```python
from build123d import *

# Parameters (mm, degrees)
PAD_DEPTH        = 44
SKETCH001_W      = 79.5
SKETCH001_H      = 39.5
POCKET_DEPTH     = 42
SKETCH003_W      = 79.5
SKETCH003_H      = 39.5
PAD001_DEPTH     = 11
SKETCH004_W      = 75.5
SKETCH004_H      = 35.5
POCKET001_DEPTH  = 11
HOLE_D           = 5.3
HOLE_DEPTH       = 25
HOLE_CSINK_D     = 6.1
HOLE_CSINK_ANGLE = 90
HOLE_TIPS_R      = 2.65
SKETCH056_W      = 7
SKETCH056_H      = 30
POCKET017_DEPTH  = 61.3
SKETCH054_W      = 7
SKETCH054_H      = 30
POCKET019_DEPTH  = 61.3
SKETCH057_W      = 12
SKETCH057_H      = 40
POCKET018_DEPTH  = 31
SKETCH055_W      = 12
SKETCH055_H      = 40
POCKET020_DEPTH  = 31
SKETCH005_W      = 15
SKETCH005_H      = 10
POCKET002_DEPTH  = 5
SKETCH058_W      = 81.5
SKETCH058_H      = 41.5
POCKET021_DEPTH  = 2
CHAMFER_SIZE     = 0.5
CHAMFER030_SIZE  = 0.3
CHAMFER031_SIZE  = 0.3


with BuildPart() as part:
    # Sketch → Pad (new body)
    with BuildSketch(Plane.XZ):
        with BuildLine():
            Line((99, 14), (99, -6))
            ThreePointArc((99, -6), (70.300448, -3.42122), (41.5, -2.5))
            Line((41.5, -21.5), (41.5, -2.5))
            ThreePointArc((-41.5, -21.5), (0, -23.225226), (41.5, -21.5))
            Line((-41.5, -2.5), (-41.5, -21.5))
            ThreePointArc((-41.5, -2.5), (-70.300448, -3.42122), (-99, -6))
            Line((-99, 14), (-99, -6))
            ThreePointArc((99, 14), (0, 23.89899), (-99, 14))
        make_face()
    extrude(amount=PAD_DEPTH)

    # Sketch001 (on DatumPlane) → Pocket (cut)
    with BuildSketch(Plane(origin=(0, 0, 0), x_dir=(1, 0, 0), z_dir=(0, 1, 0))):
        Rectangle(SKETCH001_W, SKETCH001_H)
    extrude(amount=-POCKET_DEPTH, mode=Mode.SUBTRACT)

    # Sketch003 → Pad001 (join)
    with BuildSketch(Plane(origin=(0, -42, 0), x_dir=(1, 0, 0), z_dir=(0, 1, 0))):
        Rectangle(SKETCH003_W, SKETCH003_H)
    extrude(amount=PAD001_DEPTH)

    # Sketch004 (on Face15 of Pad001) → Pocket001 (cut)
    with BuildSketch(Plane(origin=(0, -31, 0), x_dir=(1, 0, 0), z_dir=(0, 1, 0))):
        Rectangle(SKETCH004_W, SKETCH004_H)
    extrude(amount=-POCKET001_DEPTH, mode=Mode.SUBTRACT)

    # Hole
    with Locations(Plane.XZ.offset(44)):
        with Locations((-15.24, 11.43), (-7.62, 11.43), (0, 11.43), (7.62, 11.43), (15.24, 11.43), (-15.24, 3.81), (-7.62, 3.81), (0, 3.81), (7.62, 3.81), (15.24, 3.81), (-15.24, -3.81), (-7.62, -3.81), (0, -3.81), (7.62, -3.81), (15.24, -3.81), (-15.24, -11.43), (-7.62, -11.43), (0, -11.43), (7.62, -11.43), (15.24, -11.43)):
            CounterSinkHole(HOLE_D / 2, HOLE_CSINK_D / 2, depth=HOLE_DEPTH, counter_sink_angle=HOLE_CSINK_ANGLE)

    # Hole tips → Hole tip 1 section 0
    with BuildSketch(Plane.XZ.offset(19), mode=Mode.PRIVATE) as hole_tip_1_s0:
        with Locations((-15.24, 11.43)):
            Circle(HOLE_TIPS_R)
    loft([hole_tip_1_s0.sketch, Vertex(-15.24, -17.407719, 11.43)], mode=Mode.SUBTRACT)

    # Hole tips → Hole tip 2 section 0
    with BuildSketch(Plane.XZ.offset(19), mode=Mode.PRIVATE) as hole_tip_2_s0:
        with Locations((-7.62, 11.43)):
            Circle(HOLE_TIPS_R)
    loft([hole_tip_2_s0.sketch, Vertex(-7.62, -17.407719, 11.43)], mode=Mode.SUBTRACT)

    # Hole tips → Hole tip 3 section 0
    with BuildSketch(Plane.XZ.offset(19), mode=Mode.PRIVATE) as hole_tip_3_s0:
        with Locations((0, 11.43)):
            Circle(HOLE_TIPS_R)
    loft([hole_tip_3_s0.sketch, Vertex(0, -17.407719, 11.43)], mode=Mode.SUBTRACT)

    # Hole tips → Hole tip 4 section 0
    with BuildSketch(Plane.XZ.offset(19), mode=Mode.PRIVATE) as hole_tip_4_s0:
        with Locations((7.62, 11.43)):
            Circle(HOLE_TIPS_R)
    loft([hole_tip_4_s0.sketch, Vertex(7.62, -17.407719, 11.43)], mode=Mode.SUBTRACT)

    # Hole tips → Hole tip 5 section 0
    with BuildSketch(Plane.XZ.offset(19), mode=Mode.PRIVATE) as hole_tip_5_s0:
        with Locations((15.24, 11.43)):
            Circle(HOLE_TIPS_R)
    loft([hole_tip_5_s0.sketch, Vertex(15.24, -17.407719, 11.43)], mode=Mode.SUBTRACT)

    # Hole tips → Hole tip 6 section 0
    with BuildSketch(Plane.XZ.offset(19), mode=Mode.PRIVATE) as hole_tip_6_s0:
        with Locations((-15.24, 3.81)):
            Circle(HOLE_TIPS_R)
    loft([hole_tip_6_s0.sketch, Vertex(-15.24, -17.407719, 3.81)], mode=Mode.SUBTRACT)

    # Hole tips → Hole tip 7 section 0
    with BuildSketch(Plane.XZ.offset(19), mode=Mode.PRIVATE) as hole_tip_7_s0:
        with Locations((-7.62, 3.81)):
            Circle(HOLE_TIPS_R)
    loft([hole_tip_7_s0.sketch, Vertex(-7.62, -17.407719, 3.81)], mode=Mode.SUBTRACT)

    # Hole tips → Hole tip 8 section 0
    with BuildSketch(Plane.XZ.offset(19), mode=Mode.PRIVATE) as hole_tip_8_s0:
        with Locations((0, 3.81)):
            Circle(HOLE_TIPS_R)
    loft([hole_tip_8_s0.sketch, Vertex(0, -17.407719, 3.81)], mode=Mode.SUBTRACT)

    # Hole tips → Hole tip 9 section 0
    with BuildSketch(Plane.XZ.offset(19), mode=Mode.PRIVATE) as hole_tip_9_s0:
        with Locations((7.62, 3.81)):
            Circle(HOLE_TIPS_R)
    loft([hole_tip_9_s0.sketch, Vertex(7.62, -17.407719, 3.81)], mode=Mode.SUBTRACT)

    # Hole tips → Hole tip 10 section 0
    with BuildSketch(Plane.XZ.offset(19), mode=Mode.PRIVATE) as hole_tip_10_s0:
        with Locations((15.24, 3.81)):
            Circle(HOLE_TIPS_R)
    loft([hole_tip_10_s0.sketch, Vertex(15.24, -17.407719, 3.81)], mode=Mode.SUBTRACT)

    # Hole tips → Hole tip 11 section 0
    with BuildSketch(Plane.XZ.offset(19), mode=Mode.PRIVATE) as hole_tip_11_s0:
        with Locations((-15.24, -3.81)):
            Circle(HOLE_TIPS_R)
    loft([hole_tip_11_s0.sketch, Vertex(-15.24, -17.407719, -3.81)], mode=Mode.SUBTRACT)

    # Hole tips → Hole tip 12 section 0
    with BuildSketch(Plane.XZ.offset(19), mode=Mode.PRIVATE) as hole_tip_12_s0:
        with Locations((-7.62, -3.81)):
            Circle(HOLE_TIPS_R)
    loft([hole_tip_12_s0.sketch, Vertex(-7.62, -17.407719, -3.81)], mode=Mode.SUBTRACT)

    # Hole tips → Hole tip 13 section 0
    with BuildSketch(Plane.XZ.offset(19), mode=Mode.PRIVATE) as hole_tip_13_s0:
        with Locations((0, -3.81)):
            Circle(HOLE_TIPS_R)
    loft([hole_tip_13_s0.sketch, Vertex(0, -17.407719, -3.81)], mode=Mode.SUBTRACT)

    # Hole tips → Hole tip 14 section 0
    with BuildSketch(Plane.XZ.offset(19), mode=Mode.PRIVATE) as hole_tip_14_s0:
        with Locations((7.62, -3.81)):
            Circle(HOLE_TIPS_R)
    loft([hole_tip_14_s0.sketch, Vertex(7.62, -17.407719, -3.81)], mode=Mode.SUBTRACT)

    # Hole tips → Hole tip 15 section 0
    with BuildSketch(Plane.XZ.offset(19), mode=Mode.PRIVATE) as hole_tip_15_s0:
        with Locations((15.24, -3.81)):
            Circle(HOLE_TIPS_R)
    loft([hole_tip_15_s0.sketch, Vertex(15.24, -17.407719, -3.81)], mode=Mode.SUBTRACT)

    # Hole tips → Hole tip 16 section 0
    with BuildSketch(Plane.XZ.offset(19), mode=Mode.PRIVATE) as hole_tip_16_s0:
        with Locations((-15.24, -11.43)):
            Circle(HOLE_TIPS_R)
    loft([hole_tip_16_s0.sketch, Vertex(-15.24, -17.407719, -11.43)], mode=Mode.SUBTRACT)

    # Hole tips → Hole tip 17 section 0
    with BuildSketch(Plane.XZ.offset(19), mode=Mode.PRIVATE) as hole_tip_17_s0:
        with Locations((-7.62, -11.43)):
            Circle(HOLE_TIPS_R)
    loft([hole_tip_17_s0.sketch, Vertex(-7.62, -17.407719, -11.43)], mode=Mode.SUBTRACT)

    # Hole tips → Hole tip 18 section 0
    with BuildSketch(Plane.XZ.offset(19), mode=Mode.PRIVATE) as hole_tip_18_s0:
        with Locations((0, -11.43)):
            Circle(HOLE_TIPS_R)
    loft([hole_tip_18_s0.sketch, Vertex(0, -17.407719, -11.43)], mode=Mode.SUBTRACT)

    # Hole tips → Hole tip 19 section 0
    with BuildSketch(Plane.XZ.offset(19), mode=Mode.PRIVATE) as hole_tip_19_s0:
        with Locations((7.62, -11.43)):
            Circle(HOLE_TIPS_R)
    loft([hole_tip_19_s0.sketch, Vertex(7.62, -17.407719, -11.43)], mode=Mode.SUBTRACT)

    # Hole tips → Hole tip 20 section 0
    with BuildSketch(Plane.XZ.offset(19), mode=Mode.PRIVATE) as hole_tip_20_s0:
        with Locations((15.24, -11.43)):
            Circle(HOLE_TIPS_R)
    loft([hole_tip_20_s0.sketch, Vertex(15.24, -17.407719, -11.43)], mode=Mode.SUBTRACT)

    # Sketch056 → Pocket017 (cut)
    with BuildSketch(Plane(origin=(99, 0, 0), x_dir=(0, 0, 1), z_dir=(1, 0, 0))):
        with Locations((4, 22)):
            Rectangle(SKETCH056_W, SKETCH056_H)
    extrude(amount=-POCKET017_DEPTH, mode=Mode.SUBTRACT)

    # Sketch054 (on Face3 of Pocket) → Pocket019 (cut)
    with BuildSketch(Plane(origin=(-99, 0, 0), x_dir=(0, 0, -1), z_dir=(-1, 0, 0))):
        with Locations((-4, 22)):
            Rectangle(SKETCH054_W, SKETCH054_H)
    extrude(amount=-POCKET019_DEPTH, mode=Mode.SUBTRACT)

    # Sketch057 (on Face2 of Pocket017) → Pocket018 (cut)
    with BuildSketch(Plane(origin=(99, 0, 0), x_dir=(0, 0, 1), z_dir=(1, 0, 0))):
        with Locations((4, 22)):
            Rectangle(SKETCH057_W, SKETCH057_H)
    extrude(amount=-POCKET018_DEPTH, mode=Mode.SUBTRACT)

    # Sketch055 → Pocket020 (cut)
    with BuildSketch(Plane(origin=(-99, 0, 0), x_dir=(0, 0, -1), z_dir=(-1, 0, 0))):
        with Locations((-4, 22)):
            Rectangle(SKETCH055_W, SKETCH055_H)
    extrude(amount=-POCKET020_DEPTH, mode=Mode.SUBTRACT)

    # Sketch005 → Pocket002 (cut)
    with BuildSketch(Plane(origin=(0, 0, -19.75), x_dir=(-1, 0, 0), z_dir=(0, 0, 1))):
        with Locations((-3, 13)):
            Rectangle(SKETCH005_W, SKETCH005_H)
    extrude(amount=-POCKET002_DEPTH, mode=Mode.SUBTRACT)

    # Sketch058 (on Face4 of Pocket002) → Pocket021 (cut)
    with BuildSketch(Plane(origin=(0, 0, 0), x_dir=(1, 0, 0), z_dir=(0, 1, 0))):
        Rectangle(SKETCH058_W, SKETCH058_H)
    extrude(amount=-POCKET021_DEPTH, mode=Mode.SUBTRACT)

    # Chamfer
    chamfer_edges = [part.edges().sort_by_distance(p)[0] for p in [
        (70.300448, 0, -3.42122),
        (41.5, 0, -12),
        (0, 0, -23.225226),
        (-41.5, 0, -12),
        (-70.300448, 0, -3.42122),
        (0, 0, 23.89899),
        (0, -44, 23.89899),
        (-70.300448, -44, -3.42122),
        (70.300448, -44, -3.42122),
        (0, -44, -23.225226),
        (41.5, -44, -12),
        (-41.5, -44, -12),
    ]]
    chamfer(chamfer_edges, length=CHAMFER_SIZE)

    # Chamfer030
    chamfer030_edges = [part.edges().sort_by_distance(p)[0] for p in [
        (-99, -22, 10),
        (-99, -2, 4),
        (-99, -22, -2),
        (-99, -42, 4),
        (99, -22, 10),
        (99, -42, 4),
        (99, -22, -2),
        (99, -2, 4),
        (0, -2, 19.75),
        (-39.75, -2, 0),
        (0, -2, -19.75),
        (39.75, -2, 0),
    ]]
    chamfer(chamfer030_edges, length=CHAMFER030_SIZE)

    # Chamfer031
    chamfer031_edges = [part.edges().sort_by_distance(p)[0] for p in [
        (3, -18, -19.75),
        (10.5, -13, -19.75),
        (3, -8, -19.75),
        (-4.5, -13, -19.75),
        (3.000338, -18, -23.216224),
        (10.5, -13, -23.114964),
        (-4.5, -13, -23.204976),
        (3.000338, -8, -23.216224),
    ]]
    chamfer(chamfer031_edges, length=CHAMFER031_SIZE)


solid = part.part
```
Geometry: final body of the model. Coordinates: model frame, mm. A direction names the side the tool comes from. Round coordinates to 2 decimals unless told otherwise and drop trailing zeros. Use one line per item in the form item = value. Start each with the question number.
1. Line query: probe 1 along X at (y, z) = (-42.75, 3.81); probe 2 along X at (y, z) = (-17, -8.5); probe 3 along Z at (x, y) = (22, -6). Output: solid intervals per line, ascending.
2. Draft query along Z for faces 5 (the face through (-17.69, -42.79, 2.8)), 6 (the face through (1.395, -21.699, 23.897)), 7 (the face through (-99, -22, -3)). Return one class per face: pulls with the +Z half, pulls with the -Z half, needs draft (parallel to the pull), parting line crosses it, or undercut.
3. Cut plane B-B (z = -11.43). Count the separate pieces of the cut face and the enclosed holes in it, then the cut area to 3 significant figures.
4. Reachability of faces 1 (the face through (-53, -37, 4)), 2 (the face through (-84, -2, 4)), 3 (the face through (84, -22, -2)), 4 (the face through (-1, -16, 19.75)) from +Z, -Z, +X, -X, +Y, -Y: full face, straight path, thin tool, end or side. Return the list, or none.
5. Pin query (flat end, axial travel): pin 1 Ø10 at (x, y) = (32, -34.5) entering from -Z; pin 2 Ø6 at (x, z) = (76, -2) entering from +Y; pin 3 Ø5 at (x, z) = (4.5, 13) entering from +Y; pin 4 Ø4 at (y, z) = (-6, -9) entering from +X. Return the tip coordinate at first contact, or that it passes through.
Solution:
q1.probe_1 = -99 to -17.89, -12.59 to -10.27, -4.97 to -2.65, 2.65 to 4.97, 10.27 to 12.59, 17.89 to 99
q1.probe_2 = -41.5 to -39.75, 39.75 to 41.5
q1.probe_3 = -22.74 to -19.75, 19.75 to 23.41
q2.face_5 = undercut
q2.face_6 = pulls with the +Z half
q2.face_7 = needs draft
q3.separate_pieces = 6
q3.enclosed_holes = 0
q3.area = 299 mm^2
q4.face_1 = +X, -X
q4.face_2 = -X
q4.face_3 = +X
q4.face_4 = +Y
q5.pin_1 = -22.5
q5.pin_2 = 0
q5.pin_3 = -42
q5.pin_4 = 41.5
